Here's how the part is built. I have some questions about the finished solid (model axes, mm). Face numbers are marked on the shaded views. A direction names the side the tool comes from. Round coordinates to 2 decimals unless told otherwise and drop trailing zeros. Loops run counter-clockwise (first coordinate to the right, second up) from the corner with the lowest first, then second, coordinate; pieces in that order, holes last. Notation, with made-up numbers: M 57.25,86.25 L 116.25,86.25 A27 ccw 116.25,107.25 Z; hole C 36,-2.5 d4. An arc over 180 degrees is marked long. Answer as a JSON object with one key per item and string values.
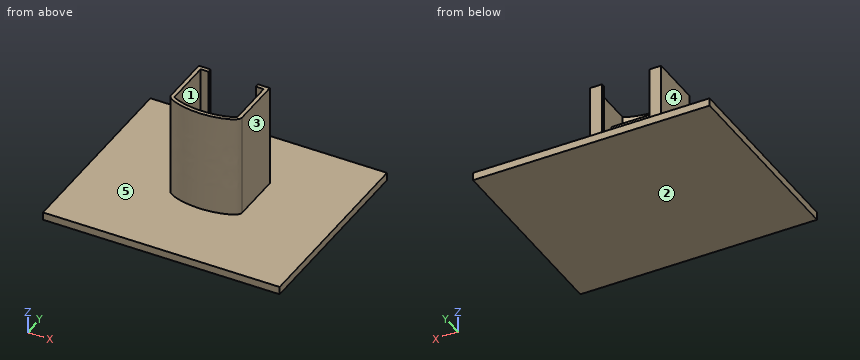
from build123d import *

# Parameters (mm, degrees)
F1_DEPTH = 26
F2_W     = 60
F2_H     = 50
F3_DEPTH = 2
F4_DEPTH = 20


with BuildPart() as f1:
    # F0 (on Top) → F1 (new body)
    with BuildSketch(Plane.XY):
        with BuildLine():
            Line((-9, 9), (-9, 0))
            Line((-9, 0), (-9, -3))
            add(Edge.make_bspline(
                [(-9, -3), (-9, -2.5707676204), (-8.6315191286, -2.1415352408), (-8, -1.7474503993)],
                knots=[0, 0, 0, 0, 0.0715387299, 0.0715387299, 0.0715387299, 0.0715387299], degree=3))
            Line((-8, -1.7474503993), (-8, 0))
            Line((-8, 0), (-8, 1))
            Line((-8, 1), (-8, 8))
            Line((-8, 8), (-6, 8))
            Line((-6, 8), (-6, 9))
            Line((-6, 9), (-9, 9))
        make_face()
        with BuildLine():
            add(Edge.make_bspline(
                [(-9, -3), (-9, -2.5707676204), (-8.6315191286, -2.1415352408), (-8, -1.7474503993)],
                knots=[0, 0, 0, 0, 0.0715387299, 0.0715387299, 0.0715387299, 0.0715387299], degree=3))
            add(Edge.make_bspline(
                [(-8.8381918042, -3.5), (-8.9439804927, -3.3347222947), (-9, -3.1673611473), (-9, -3)],
                knots=[0.9721064754, 0.9721064754, 0.9721064754, 0.9721064754, 1, 1, 1, 1], degree=3))
            add(Edge.make_bspline(
                [(-8, -2.7474503993), (-8.3852847555, -2.9878784004), (-8.6726634562, -3.2413887449), (-8.8381918042, -3.5)],
                knots=[0.9284612701, 0.9284612701, 0.9284612701, 0.9284612701, 0.9721064754, 0.9721064754, 0.9721064754, 0.9721064754], degree=3))
            Line((-8, -2.7474503993), (-8, -1.7474503993))
        make_face()
        with BuildLine():
            add(Edge.make_bspline(
                [(-8.8381918042, -3.5), (-8.9439804927, -3.3347222947), (-9, -3.1673611473), (-9, -3)],
                knots=[0.9721064754, 0.9721064754, 0.9721064754, 0.9721064754, 1, 1, 1, 1], degree=3))
            Line((-9, -3), (-9, -4))
            add(Edge.make_bspline(
                [(-8.8381918042, -3.5), (-8.9439804927, -3.6652777053), (-9, -3.8326388527), (-9, -4)],
                knots=[0.9721064754, 0.9721064754, 0.9721064754, 0.9721064754, 1, 1, 1, 1], degree=3))
        make_face()
        with BuildLine():
            add(Edge.make_bspline(
                [(-8, -2.7474503993), (-8.3852847555, -2.9878784004), (-8.6726634562, -3.2413887449), (-8.8381918042, -3.5)],
                knots=[0.9284612701, 0.9284612701, 0.9284612701, 0.9284612701, 0.9721064754, 0.9721064754, 0.9721064754, 0.9721064754], degree=3))
            add(Edge.make_bspline(
                [(-8, -4.2525496007), (-8.3852847555, -4.0121215996), (-8.6726634562, -3.7586112551), (-8.8381918042, -3.5)],
                knots=[0.9284612701, 0.9284612701, 0.9284612701, 0.9284612701, 0.9721064754, 0.9721064754, 0.9721064754, 0.9721064754], degree=3))
            Line((-8, -4.2525496007), (-8, -2.7474503993))
        make_face()
        with BuildLine():
            add(Edge.make_bspline(
                [(-8.8381918042, -3.5), (-8.9439804927, -3.6652777053), (-9, -3.8326388527), (-9, -4)],
                knots=[0.9721064754, 0.9721064754, 0.9721064754, 0.9721064754, 1, 1, 1, 1], degree=3))
            add(Edge.make_bspline(
                [(-9, -4), (-9, -5.5), (0, -8.5), (9, -5.5), (9, -4)],
                knots=[0, 0, 0, 0, 0.25, 0.5, 0.5, 0.5, 0.5], degree=3))
            add(Edge.make_bspline(
                [(9, -4), (9, -3.8326388527), (8.9439804927, -3.6652777053), (8.8381918042, -3.5)],
                knots=[0.5, 0.5, 0.5, 0.5, 0.5278935246, 0.5278935246, 0.5278935246, 0.5278935246], degree=3))
            add(Edge.make_bspline(
                [(8.8381918042, -3.5), (8.6726634562, -3.7586112551), (8.3852847555, -4.0121215996), (8, -4.2525496007)],
                knots=[0.5278935246, 0.5278935246, 0.5278935246, 0.5278935246, 0.5715387299, 0.5715387299, 0.5715387299, 0.5715387299], degree=3))
            add(Edge.make_bspline(
                [(8, -4.2525496007), (6.4246057224, -5.2356378021), (0, -6.7643621979), (-6.4246057224, -5.2356378021), (-8, -4.2525496007)],
                knots=[0.5715387299, 0.5715387299, 0.5715387299, 0.5715387299, 0.75, 0.9284612701, 0.9284612701, 0.9284612701, 0.9284612701], degree=3))
            add(Edge.make_bspline(
                [(-8, -4.2525496007), (-8.3852847555, -4.0121215996), (-8.6726634562, -3.7586112551), (-8.8381918042, -3.5)],
                knots=[0.9284612701, 0.9284612701, 0.9284612701, 0.9284612701, 0.9721064754, 0.9721064754, 0.9721064754, 0.9721064754], degree=3))
        make_face()
        with BuildLine():
            add(Edge.make_bspline(
                [(8.8381918042, -3.5), (8.6726634562, -3.7586112551), (8.3852847555, -4.0121215996), (8, -4.2525496007)],
                knots=[0.5278935246, 0.5278935246, 0.5278935246, 0.5278935246, 0.5715387299, 0.5715387299, 0.5715387299, 0.5715387299], degree=3))
            add(Edge.make_bspline(
                [(8.8381918042, -3.5), (8.6726634562, -3.2413887449), (8.3852847555, -2.9878784004), (8, -2.7474503993)],
                knots=[0.5278935246, 0.5278935246, 0.5278935246, 0.5278935246, 0.5715387299, 0.5715387299, 0.5715387299, 0.5715387299], degree=3))
            Line((8, -2.7474503993), (8, -4.2525496007))
        make_face()
        with BuildLine():
            add(Edge.make_bspline(
                [(9, -3), (9, -3.1673611473), (8.9439804927, -3.3347222947), (8.8381918042, -3.5)],
                knots=[0.5, 0.5, 0.5, 0.5, 0.5278935246, 0.5278935246, 0.5278935246, 0.5278935246], degree=3))
            add(Edge.make_bspline(
                [(8, -1.7474503993), (8.6315191286, -2.1415352408), (9, -2.5707676204), (9, -3)],
                knots=[0.4284612701, 0.4284612701, 0.4284612701, 0.4284612701, 0.5, 0.5, 0.5, 0.5], degree=3))
            Line((8, -1.7474503993), (8, -2.7474503993))
            add(Edge.make_bspline(
                [(8.8381918042, -3.5), (8.6726634562, -3.2413887449), (8.3852847555, -2.9878784004), (8, -2.7474503993)],
                knots=[0.5278935246, 0.5278935246, 0.5278935246, 0.5278935246, 0.5715387299, 0.5715387299, 0.5715387299, 0.5715387299], degree=3))
        make_face()
        with BuildLine():
            add(Edge.make_bspline(
                [(8, -1.7474503993), (8.6315191286, -2.1415352408), (9, -2.5707676204), (9, -3)],
                knots=[0.4284612701, 0.4284612701, 0.4284612701, 0.4284612701, 0.5, 0.5, 0.5, 0.5], degree=3))
            Line((9, -3), (9, 0))
            Line((9, 0), (9, 9))
            Line((9, 9), (6, 9))
            Line((6, 9), (6, 8))
            Line((6, 8), (8, 8))
            Line((8, 8), (8, 1))
            Line((8, 1), (8, 0))
            Line((8, 0), (8, -1.7474503993))
        make_face()
        with BuildLine():
            add(Edge.make_bspline(
                [(9, -4), (9, -3.8326388527), (8.9439804927, -3.6652777053), (8.8381918042, -3.5)],
                knots=[0.5, 0.5, 0.5, 0.5, 0.5278935246, 0.5278935246, 0.5278935246, 0.5278935246], degree=3))
            Line((9, -4), (9, -3))
            add(Edge.make_bspline(
                [(9, -3), (9, -3.1673611473), (8.9439804927, -3.3347222947), (8.8381918042, -3.5)],
                knots=[0.5, 0.5, 0.5, 0.5, 0.5278935246, 0.5278935246, 0.5278935246, 0.5278935246], degree=3))
        make_face()
    extrude(amount=F1_DEPTH)

    # F2 (on Top) → F3 (join)
    with BuildSketch(Plane.XY):
        Rectangle(F2_W, F2_H)
    extrude(amount=-F3_DEPTH)

    # F0 (on Top) → F4 (join)
    with BuildSketch(Plane.XY):
        Polygon((-8, 0), (0, 0), (8, 0), (8, 1), (-8, 1), align=None)
    extrude(amount=F4_DEPTH)


solid = f1.part
Item 1: For P1, Ø0.5, axis at y = 8.5, z = 10.5, coming from the +X side; P2, Ø13.5, axis at y = 2.5, z = 10, coming from the -X side; P3, Ø3, axis at x = -19, y = -19, coming from the +Z side; P4, Ø12, axis at y = 16, z = 14, coming from the +X side, each with a flat end and sliding along its axis, tell me the tip position at first contact or that it passes through.
Solution:
{"P1": "stops at x = 9", "P2": "stops at x = -9", "P3": "stops at z = 0", "P4": "passes through"}
Item 2: I want a section at A-A on y = 6. List the corners of the cut face in (x, z) for me.
Solution:
{"outline": "M -30,-2 L 30,-2 L 30,0 L 9,0 L 9,26 L 8,26 L 8,0 L -8,0 L -8,26 L -9,26 L -9,0 L -30,0 Z"}
Item 3: If I drill on L1, parallel to X at y = 6.5, z = 23.5; L2, parallel to Z at x = -23, y = 1.5; L3, parallel to Y at x = -3, z = 4, over which ranges is the centre line in solid material (lowest first)? Write a range as from..to.
Solution:
{"L1": "x = -9..-8, 8..9", "L2": "z = -2..0", "L3": "y = -6.79..-5.79, 0..1"}
Item 4: For the marked faces 4 and 5, which set-ups out of +Z, -Z, +X, -X, +Y, -Y let a thin tool reach every point of the face, with its end or its side?
Solution:
{"face 4": "+Z, -X, +Y, -Y", "face 5": "+Z"}
Item 5: We'd pull the mould along X, two halves only. Please class the marked faces 1, 2 and 3: +X half, -X half, draft (parallel to the pull), parting line (faces both ways), or undercut.
Solution:
{"face 1": "undercut", "face 2": "draft", "face 3": "+X half"}
Item 6: I want a section at B-B on x = 20. List the corners of the cut face in (y, z) for me, plus the area to 3 significant figures.
Solution:
{"outline": "M -25,-2 L 25,-2 L 25,0 L -25,0 Z", "area": "100 mm2"}
